Check sheet for the modelled part. Datum: model origin and axes. Units: mm. A direction names the side the tool comes from. Coordinates: 2 decimals unless noted, no trailing zeros. Loops run counter-clockwise (first coordinate to the right, second up) from the corner with the lowest first, then second, coordinate; pieces in that order, holes last. Notation, with made-up numbers: M 11.5,-26 L 52.5,-26 A13 cw 52.5,-13 Z; hole C -2.75,20.25 d6. An arc over 180 degrees is marked long. Answer as CSV lines item,"result". Start each with the question number.
from build123d import *

# Parameters (mm, degrees)
F0_R          = 1.25
F0_R_2        = 12
F1_DEPTH      = 5
F0_R_3        = 1
F2_START      = 3
F0_R_4        = 2
F2_DEPTH      = 2
F4_START      = 1.6
F4_DEPTH      = 3.4
F5_DEPTH      = 1.3
F5_DEPTH_BACK = 0.1


# Not quite as in the source:
# - a feature of the source that left no trace in its solid (it failed there, or was rolled back) is left out


with BuildPart() as f1:
    # F0 (on Top) → F1 (new body)
    with BuildSketch(Plane.XY):
        with BuildLine():
            Line((6.0037070689, 60.0215111673), (-5, 60.0215111673))
            Line((-5, 60.0215111673), (-6.7870675903, 60.0215111673))
            ThreePointArc((-6.7870675903, 60.0215111673), (-12.5859769766, 57.1353808627), (-15, 51.1245913098))
            Line((-15, 51.1245913098), (-15, 50.7903024554))
            Line((-15, 50.7903024554), (-15, -49.5038591325))
            Line((-15, -49.5038591325), (-15, -51.7690908138))
            ThreePointArc((-15, -51.7690908138), (-12.1695256151, -57.4125609321), (-6.4009595691, -59.9784888327))
            Line((-6.4009595691, -59.9784888327), (-5, -59.9784888327))
            Line((-5, -59.9784888327), (5, -59.9784888327))
            Line((5, -59.9784888327), (7.0074141379, -59.9784888327))
            ThreePointArc((7.0074141379, -59.9784888327), (12.2930504345, -57.5138166091), (15, -52.3480655233))
            Line((15, -52.3480655233), (15, -49.5038591325))
            Line((15, -49.5038591325), (15, 50.7903024554))
            Line((15, 50.7903024554), (15, 50.95497525))
            ThreePointArc((15, 50.95497525), (12.3454627339, 57.317569046), (6.0037070689, 60.0215111673))
        make_face()
        with Locations((-9.525, -56.2587864697)):
            Circle(F0_R, mode=Mode.SUBTRACT)
        with Locations((-9.525, -30.4671674967)):
            Circle(F0_R, mode=Mode.SUBTRACT)
        with Locations((0, -44.7514858243)):
            Circle(F0_R_2, mode=Mode.SUBTRACT)
        with Locations((-9.525, 0)):
            Circle(F0_R, mode=Mode.SUBTRACT)
        with Locations((0, -15.4157546586)):
            Circle(F0_R_2, mode=Mode.SUBTRACT)
        with Locations((9.525, -56.2587864697)):
            Circle(F0_R, mode=Mode.SUBTRACT)
        with Locations((9.525, -30.4671674967)):
            Circle(F0_R, mode=Mode.SUBTRACT)
        with Locations((9.525, 0)):
            Circle(F0_R, mode=Mode.SUBTRACT)
        with Locations((-9.525, 29.1974432766)):
            Circle(F0_R, mode=Mode.SUBTRACT)
        with Locations((0, 15.3948861798)):
            Circle(F0_R_2, mode=Mode.SUBTRACT)
        with Locations((-9.525, 55.7628124952)):
            Circle(F0_R, mode=Mode.SUBTRACT)
        with Locations((0, 44.3624239764)):
            Circle(F0_R_2, mode=Mode.SUBTRACT)
        with Locations((9.525, 29.1974432766)):
            Circle(F0_R, mode=Mode.SUBTRACT)
        with Locations((9.525, 55.7628124952)):
            Circle(F0_R, mode=Mode.SUBTRACT)
        with BuildLine():
            ThreePointArc((15, 50.7903024554), (15.0003704536, 50.8726388527), (15, 50.95497525))
            Line((15, 50.95497525), (15, 50.7903024554))
        make_face()
    extrude(amount=F1_DEPTH)



with BuildPart() as f1b:
    # F0 (on Top) → F1, piece 2 (new body)
    with BuildSketch(Plane.XY):
        with Locations((-9.525, 44.3624239764)):
            Circle(F0_R_3)
    extrude(amount=F1_DEPTH)


with BuildPart() as f1c:
    # F0 (on Top) → F1, piece 3 (new body)
    with BuildSketch(Plane.XY):
        with Locations((9.525, 44.3624239764)):
            Circle(F0_R_3)
    extrude(amount=F1_DEPTH)


with BuildPart() as f1d:
    # F0 (on Top) → F1, piece 4 (new body)
    with BuildSketch(Plane.XY):
        with Locations((9.525, 15.3948861798)):
            Circle(F0_R_3)
    extrude(amount=F1_DEPTH)


with BuildPart() as f1e:
    # F0 (on Top) → F1, piece 5 (new body)
    with BuildSketch(Plane.XY):
        with Locations((-9.525, 15.3948861798)):
            Circle(F0_R_3)
    extrude(amount=F1_DEPTH)


with BuildPart() as f1f:
    # F0 (on Top) → F1, piece 6 (new body)
    with BuildSketch(Plane.XY):
        with Locations((9.525, -15.4157546586)):
            Circle(F0_R_3)
    extrude(amount=F1_DEPTH)


with BuildPart() as f1g:
    # F0 (on Top) → F1, piece 7 (new body)
    with BuildSketch(Plane.XY):
        with Locations((-9.525, -15.4157546586)):
            Circle(F0_R_3)
    extrude(amount=F1_DEPTH)


with BuildPart() as f1h:
    # F0 (on Top) → F1, piece 8 (new body)
    with BuildSketch(Plane.XY):
        with Locations((9.525, -44.7514858243)):
            Circle(F0_R_3)
    extrude(amount=F1_DEPTH)


with BuildPart() as f1i:
    # F0 (on Top) → F1, piece 9 (new body)
    with BuildSketch(Plane.XY):
        with Locations((-9.525, -44.7514858243)):
            Circle(F0_R_3)
    extrude(amount=F1_DEPTH)


with BuildPart() as f1_1:
    add(f1.part)

    add(f1b.part)  # F2 merges F1b

    add(f1c.part)  # F2 merges F1c

    add(f1d.part)  # F2 merges F1d

    add(f1e.part)  # F2 merges F1e

    add(f1f.part)  # F2 merges F1f

    add(f1g.part)  # F2 merges F1g

    add(f1h.part)  # F2 merges F1h

    add(f1i.part)  # F2 merges F1i
    # F0 (on Top) → F2 (join)
    with BuildSketch(Plane.XY.offset(F2_START)):
        with Locations((0, 44.3624239764)):
            Circle(F0_R_2)
        with Locations((-9.525, 44.3624239764)):
            Circle(F0_R_4, mode=Mode.SUBTRACT)
        with Locations((9.525, 44.3624239764)):
            Circle(F0_R_4, mode=Mode.SUBTRACT)
        with Locations((0, 15.3948861798)):
            Circle(F0_R_2)
        with Locations((-9.525, 15.3948861798)):
            Circle(F0_R_4, mode=Mode.SUBTRACT)
        with Locations((9.525, 15.3948861798)):
            Circle(F0_R_4, mode=Mode.SUBTRACT)
        with Locations((0, -15.4157546586)):
            Circle(F0_R_2)
        with Locations((-9.525, -15.4157546586)):
            Circle(F0_R_4, mode=Mode.SUBTRACT)
        with Locations((9.525, -15.4157546586)):
            Circle(F0_R_4, mode=Mode.SUBTRACT)
        with Locations((0, -44.7514858243)):
            Circle(F0_R_2)
        with Locations((-9.525, -44.7514858243)):
            Circle(F0_R_4, mode=Mode.SUBTRACT)
        with Locations((9.525, -44.7514858243)):
            Circle(F0_R_4, mode=Mode.SUBTRACT)
        with Locations((9.525, 44.3624239764)):
            Circle(F0_R_4)
        with Locations((9.525, 44.3624239764)):
            Circle(F0_R_3, mode=Mode.SUBTRACT)
        with Locations((-9.525, 44.3624239764)):
            Circle(F0_R_4)
        with Locations((-9.525, 44.3624239764)):
            Circle(F0_R_3, mode=Mode.SUBTRACT)
        with Locations((9.525, 15.3948861798)):
            Circle(F0_R_4)
        with Locations((9.525, 15.3948861798)):
            Circle(F0_R_3, mode=Mode.SUBTRACT)
        with Locations((-9.525, 15.3948861798)):
            Circle(F0_R_4)
        with Locations((-9.525, 15.3948861798)):
            Circle(F0_R_3, mode=Mode.SUBTRACT)
        with Locations((9.525, -15.4157546586)):
            Circle(F0_R_4)
        with Locations((9.525, -15.4157546586)):
            Circle(F0_R_3, mode=Mode.SUBTRACT)
        with Locations((-9.525, -15.4157546586)):
            Circle(F0_R_4)
        with Locations((-9.525, -15.4157546586)):
            Circle(F0_R_3, mode=Mode.SUBTRACT)
        with Locations((9.525, -44.7514858243)):
            Circle(F0_R_4)
        with Locations((9.525, -44.7514858243)):
            Circle(F0_R_3, mode=Mode.SUBTRACT)
        with Locations((-9.525, -44.7514858243)):
            Circle(F0_R_4)
        with Locations((-9.525, -44.7514858243)):
            Circle(F0_R_3, mode=Mode.SUBTRACT)
        with Locations((9.525, -56.2587864697)):
            Circle(F0_R)
        with Locations((-9.525, -56.2587864697)):
            Circle(F0_R)
        with Locations((-9.525, -30.4671674967)):
            Circle(F0_R)
        with Locations((9.525, -30.4671674967)):
            Circle(F0_R)
        with Locations((9.525, 0)):
            Circle(F0_R)
        with Locations((-9.525, 0)):
            Circle(F0_R)
        with Locations((-9.525, 29.1974432766)):
            Circle(F0_R)
        with Locations((9.525, 29.1974432766)):
            Circle(F0_R)
        with Locations((-9.525, 55.7628124952)):
            Circle(F0_R)
        with Locations((9.525, 55.7628124952)):
            Circle(F0_R)
        with Locations((9.525, 44.3624239764)):
            Circle(F0_R_3)
        with Locations((-9.525, 44.3624239764)):
            Circle(F0_R_3)
        with Locations((9.525, 15.3948861798)):
            Circle(F0_R_3)
        with Locations((-9.525, 15.3948861798)):
            Circle(F0_R_3)
        with Locations((9.525, -15.4157546586)):
            Circle(F0_R_3)
        with Locations((-9.525, -15.4157546586)):
            Circle(F0_R_3)
        with Locations((9.525, -44.7514858243)):
            Circle(F0_R_3)
        with Locations((-9.525, -44.7514858243)):
            Circle(F0_R_3)
    extrude(amount=F2_DEPTH)

    # F0 (on Top) → F4 (join)
    with BuildSketch(Plane.XY.offset(F4_START)):
        with Locations((9.525, 44.3624239764)):
            Circle(F0_R_4)
        with Locations((9.525, 44.3624239764)):
            Circle(F0_R_3, mode=Mode.SUBTRACT)
        with Locations((-9.525, 44.3624239764)):
            Circle(F0_R_4)
        with Locations((-9.525, 44.3624239764)):
            Circle(F0_R_3, mode=Mode.SUBTRACT)
        with Locations((9.525, 15.3948861798)):
            Circle(F0_R_4)
        with Locations((9.525, 15.3948861798)):
            Circle(F0_R_3, mode=Mode.SUBTRACT)
        with Locations((-9.525, 15.3948861798)):
            Circle(F0_R_4)
        with Locations((-9.525, 15.3948861798)):
            Circle(F0_R_3, mode=Mode.SUBTRACT)
        with Locations((9.525, -15.4157546586)):
            Circle(F0_R_4)
        with Locations((9.525, -15.4157546586)):
            Circle(F0_R_3, mode=Mode.SUBTRACT)
        with Locations((-9.525, -15.4157546586)):
            Circle(F0_R_4)
        with Locations((-9.525, -15.4157546586)):
            Circle(F0_R_3, mode=Mode.SUBTRACT)
        with Locations((9.525, -44.7514858243)):
            Circle(F0_R_4)
        with Locations((9.525, -44.7514858243)):
            Circle(F0_R_3, mode=Mode.SUBTRACT)
        with Locations((-9.525, -44.7514858243)):
            Circle(F0_R_4)
        with Locations((-9.525, -44.7514858243)):
            Circle(F0_R_3, mode=Mode.SUBTRACT)
    extrude(amount=F4_DEPTH)

    # F0 (on Top) → F5 (cut, two sides)
    with BuildSketch(Plane.XY) as f5_sk:
        with Locations((9.525, -56.2587864697)):
            Circle(F0_R)
        with Locations((-9.525, -56.2587864697)):
            Circle(F0_R)
        with Locations((-9.525, -30.4671674967)):
            Circle(F0_R)
        with Locations((9.525, -30.4671674967)):
            Circle(F0_R)
        with Locations((9.525, 0)):
            Circle(F0_R)
        with Locations((-9.525, 0)):
            Circle(F0_R)
        with Locations((9.525, 29.1974432766)):
            Circle(F0_R)
        with Locations((-9.525, 29.1974432766)):
            Circle(F0_R)
        with Locations((9.525, 55.7628124952)):
            Circle(F0_R)
        with Locations((-9.525, 55.7628124952)):
            Circle(F0_R)
    extrude(amount=F5_DEPTH, mode=Mode.SUBTRACT)
    extrude(f5_sk.sketch, amount=-F5_DEPTH_BACK, mode=Mode.SUBTRACT)


solid = f1_1.part
Item 1: Material ranges on line 1 (Y direction, x = -0.5, z = 1.3); line 2 (Y direction, x = 0, z = 1.6); line 3 (X direction, y = 30, z = 2.9), recorded low to high. Write a range as from..to.
Item 2: Set-up check for faces 3 (the face through (10, -45, 0)), 4 (the face through (10.4, 43.5, 1.6)): record each of +Z, -Z, +X, -X, +Y, -Y from which the full face is reachable in a straight line by a thin tool's end or side.
Item 3: Sectioned sample at C-C, the plane x = 0. Record the boundary of the cut face in (y, z), and give its area (3 significant figures).
Item 4: Release check for a two-part mould opening along X. For faces 1 (the face through (-9.655, 45.354, 0.789)), 2 (the face through (-10, 44, 0)) record: released by +X, released by -X, zero draft, split by the parting line, or undercut.
Item 5: Go/stop test with a flat-tipped pin: pin 1 (1.5 mm diameter, centred on x = -0.5, y = -9, fed in from -Z). Record where the tip stops, or that it passes through.
Item 6: Sectioned sample at D-D, the plane y = 53.5. Record the boundary of the cut face in (x, z).
Item 7: Sectioned sample at A-A, the plane y = 0. Record the boundary of the cut face in (x, z) (3 decimals).
Item 8: Sectioned sample at B-B, the plane z = 4.2. Record the boundary of the cut face in (x, y), and give its area (3 significant figures).
Reply:
1,line 1,"-59.98..-56.74, -32.76..-27.41, -3.43..3.41, 27.38..32.37, 56.35..60.02"
1,line 2,"-59.98..-56.75, -32.75..-27.42, -3.42..3.39, 27.39..32.36, 56.36..60.02"
1,line 3,"-15..-10.48, -8.57..8.57, 10.48..15"
2,face 3,"-Z, +X, -X, +Y, -Y"
2,face 4,"-Z"
3,outline,"M -59.98,0 L -56.75,0 L -56.75,3 L -32.75,3 L -32.75,0 L -27.42,0 L -27.42,3 L -3.42,3 L -3.42,0 L 3.39,0 L 3.39,3 L 27.39,3 L 27.39,0 L 32.36,0 L 32.36,3 L 56.36,3 L 56.36,0 L 60.02,0 L 60.02,5 L -59.98,5 Z"
3,area,"312 mm²"
4,face 1,"undercut"
4,face 2,"zero draft"
5,pin 1,"z = 3"
6,outline,"M -14.64,0 L -7.78,0 L -7.78,3 L 7.78,3 L 7.78,0 L 14.62,0 L 14.62,5 L -14.64,5 Z"
7,outline,"M -15,0 L -10.775,0 L -10.775,3 L -8.275,3 L -8.275,0 L 8.275,0 L 8.275,3 L 10.775,3 L 10.775,0 L 15,0 L 15,5 L -15,5 Z"
8,outline,"M -15,-51.77 A9.37 ccw -6.4,-59.98 L 7.01,-59.98 A9.11 ccw 15,-52.35 L 15,50.79 A9.15 ccw 6,60.02 L -6.79,60.02 A9.11 ccw -15,51.12 Z"
8,area,"3,530 mm²"
